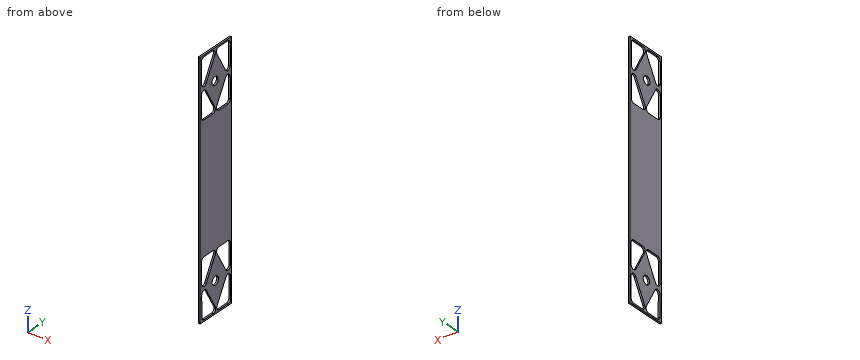
Autodesk Inventor part; units mm, degrees
ref_plane "YZ Plane" through (0, 0, 0) normal (1, 0, 0) x (0, 1, 0)
ref_plane "XZ Plane" through (0, 0, 0) normal (0, 1, 0) x (-1, 0, 0)
ref_plane "XY Plane" through (0, 0, 0) normal (0, 0, 1) x (1, 0, 0)
sketch "Sketch1" plane through (0, 0, 0) normal (1, 0, 0) x (0, 1, 0)
  line L0 (0, 0) -> (152.4, 0)
  line L1 (152.4, 0) -> (152.4, -914.4)
  line L2 (152.4, -914.4) -> (0, -914.4)
  line L3 (0, -914.4) -> (0, 0)
  dimension "d0" = 152.4
  dimension "d1" = 914.4
extrude "Extrusion1" add sketch "Sketch1" along normal blind 6.35
sketch "Sketch2" plane through (6.35, 0, 0) normal (1, 0, 0) x (0, 0, -1)
  line L0 (0, 152.4) -> (0, 0) construction
  line L1 (914.4, 152.4) -> (0, 152.4) construction
  line L2 (0, 152.4) -> (457.2, 152.4) construction
  line L3 (228.6, 152.4) -> (0, 152.4) construction
  line L4 (17.9147, 146.1725) -> (95.9969, 146.1725)
  arc A0 (101.8461, 123.5552) -> (95.9969, 146.1725) centre (95.9969, 134.1075) ccw
  line L5 (101.8461, 123.5552) -> (23.7639, 80.2737)
  arc A1 (5.8497, 90.826) -> (23.7639, 80.2737) centre (17.9147, 90.826) ccw
  line L6 (5.8497, 90.826) -> (5.8497, 134.1075)
  arc A2 (17.9147, 146.1725) -> (5.8497, 134.1075) centre (17.9147, 134.1075) ccw
  line L7 (210.6853, 146.1725) -> (132.6031, 146.1725)
  arc A3 (132.6031, 146.1725) -> (126.7539, 123.5552) centre (132.6031, 134.1075) ccw
  line L8 (126.7539, 123.5552) -> (204.8361, 80.2737)
  arc A4 (204.8361, 80.2737) -> (222.7503, 90.826) centre (210.6853, 90.826) ccw
  line L9 (222.7503, 90.826) -> (222.7503, 134.1075)
  arc A5 (222.7503, 134.1075) -> (210.6853, 146.1725) centre (210.6853, 134.1075) ccw
  line L10 (17.9147, 6.2275) -> (95.9969, 6.2275)
  arc A6 (95.9969, 6.2275) -> (101.8461, 28.8448) centre (95.9969, 18.2925) ccw
  line L11 (101.8461, 28.8448) -> (23.7639, 72.1263)
  arc A7 (23.7639, 72.1263) -> (5.8497, 61.574) centre (17.9147, 61.574) ccw
  line L12 (5.8497, 61.574) -> (5.8497, 18.2925)
  arc A8 (5.8497, 18.2925) -> (17.9147, 6.2275) centre (17.9147, 18.2925) ccw
  line L13 (126.7539, 28.8448) -> (204.8361, 72.1263)
  line L14 (210.6853, 6.2275) -> (132.6031, 6.2275)
  line L15 (222.7503, 61.574) -> (222.7503, 18.2925)
  arc A9 (222.7503, 61.574) -> (204.8361, 72.1263) centre (210.6853, 61.574) ccw
  arc A10 (210.6853, 6.2275) -> (222.7503, 18.2925) centre (210.6853, 18.2925) ccw
  arc A11 (126.7539, 28.8448) -> (132.6031, 6.2275) centre (132.6031, 18.2925) ccw
  line L16 (896.5064, 147.907) -> (818.4249, 147.5987)
  arc A12 (818.4249, 147.5987) -> (812.6651, 124.9585) centre (818.4726, 135.5338) ccw
  line L17 (812.6651, 124.9585) -> (890.9175, 81.9857)
  arc A13 (890.9175, 81.9857) -> (908.7899, 92.6086) centre (896.725, 92.561) ccw
  line L18 (908.7899, 92.6086) -> (908.619, 135.8897)
  arc A14 (908.619, 135.8897) -> (896.5064, 147.907) centre (896.5541, 135.8421) ccw
  line L19 (787.7574, 124.8602) -> (709.8468, 81.2707)
  line L20 (703.7374, 147.1459) -> (781.8189, 147.4542)
  line L21 (691.891, 91.7522) -> (691.7201, 135.0333)
  arc A15 (691.891, 91.7522) -> (709.8468, 81.2707) centre (703.9559, 91.7998) ccw
  arc A16 (703.7374, 147.1459) -> (691.7201, 135.0333) centre (703.785, 135.081) ccw
  arc A17 (787.7574, 124.8602) -> (781.8189, 147.4542) centre (781.8665, 135.3893) ccw
  arc A18 (897.059, 7.9631) -> (909.0763, 20.0757) centre (897.0113, 20.028) ccw
  line L22 (897.059, 7.9631) -> (818.9775, 7.6548)
  line L23 (813.039, 30.2488) -> (890.9496, 73.8383)
  arc A19 (813.039, 30.2488) -> (818.9775, 7.6548) centre (818.9298, 19.7197) ccw
  line L24 (908.9054, 63.3568) -> (909.0763, 20.0757)
  arc A20 (908.9054, 63.3568) -> (890.9496, 73.8383) centre (896.8405, 63.3092) ccw
  arc A21 (782.3715, 7.5103) -> (788.1313, 30.1505) centre (782.3238, 19.5752) ccw
  line L25 (704.29, 7.202) -> (782.3715, 7.5103)
  arc A22 (709.8789, 73.1233) -> (692.0065, 62.5004) centre (704.0714, 62.548) ccw
  line L26 (692.0065, 62.5004) -> (692.1774, 19.2192)
  arc A23 (692.1774, 19.2192) -> (704.29, 7.202) centre (704.2423, 19.2669) ccw
  line L27 (788.1313, 30.1505) -> (709.8789, 73.1233)
  circle A24 centre (114.3, 72.0167) radius 15.5575
  circle A25 centre (800.4147, 73.3712) radius 15.5575
extrude "Extrusion3" cut sketch "Sketch2" against normal blind 25.4
properties part number "R-SideV1"
Here's how the part is built. I have some questions about the finished solid (model axes, mm). Coordinates: 2 decimals unless noted, no trailing zeros. Loops run counter-clockwise (first coordinate to the right, second up) from the corner with the lowest first, then second, coordinate; pieces in that order, holes last. Notation, with made-up numbers: (-37.75, -37) - (-7.75, -37) arc R27 cw to (-7.75, -20) - close; hole circle Ø1 at (-21, -28.5). An arc over 180 degrees is marked (long way). Return JSON: item names as keys, results as strings. Group by question number.
Item 1: I need wall thicknesses on line 1 (Y direction, x = 4, z = -114.3); line 2 (Z direction, x = 5.5, y = 100.5); line 3 (Z direction, x = 1.5, y = 24.5). Which ranges of each line are inside material? Lowest first, please. Write a range as from..to.
Item 2: If we section it at B-B on x = 4.5: State how many separate pieces and enclosed holes the cut face has, and give its area (3 significant figures).
Item 3: If we section it at A-A on y = 47: Write out the boundary of the cut face in (x, z), and give its area (3 significant figures).
Calculated:
{
 "1": {"line 1": "y = 0..56.46, 87.57..152.4", "line 2": "z = -914.4..-908.76, -857.2..-744.22, -691.86..-222.75, -168.35..-60.25, -5.85..0", "line 3": "z = -914.4..-909.06, -807.85..-793.34, -692.16..-222.75, -122.26..-106.34, -5.85..0"},
 "2": {"separate pieces": "1", "enclosed holes": "10", "area": "100,000 mm^2"},
 "3": {"outline": "(0, -914.4) - (6.35, -914.4) - (6.35, -908.97) - (0, -908.97) - close; (0, -842.98) - (6.35, -842.98) - (6.35, -757.45) - (0, -757.45) - close; (0, -692.07) - (6.35, -692.07) - (6.35, -222.75) - (0, -222.75) - close; (0, -159.51) - (6.35, -159.51) - (6.35, -69.09) - (0, -69.09) - close; (0, -5.85) - (6.35, -5.85) - (6.35, 0) - (0, 0) - close", "area": "4,170 mm^2"}
}
